from build123d import *

# Parameters (mm, degrees)
BOSS_EXTRUDE1_DEPTH = 5.08
BOSS_EXTRUDE2_DEPTH = 8.763
CHAMFER1_SIZE       = 2.54
CUT_EXTRUDE2_DEPTH  = 6.35
SKETCH6_W           = 10.16
SKETCH6_H           = 8.89
CUT_EXTRUDE3_DEPTH  = 3.81
SKETCH7_R           = 4.953
CUT_EXTRUDE4_DEPTH  = 2.54
SKETCH8_R           = 1.786664303
SKETCH8_R_2         = 1.778
CUT_EXTRUDE5_DEPTH  = 3.54
CUT_EXTRUDE6_DEPTH  = 2.54
CUT_EXTRUDE7_DEPTH  = 0.762
SKETCH11_W          = 8.89
SKETCH11_H          = 8.89
SKETCH11_R          = 1.524
BOSS_EXTRUDE3_DEPTH = 3.175


with BuildPart() as part:
    # Sketch1 → Boss-Extrude1 (new body)
    with BuildSketch(Plane.XY):
        with BuildLine():
            Line((-12.7, 0), (-12.7, -71.267258261))
            ThreePointArc((-12.7, -71.267258261), (0, -72.39), (12.7, -71.267258261))
            Line((12.7, -71.267258261), (12.7, 0))
            Line((12.7, 0), (-12.7, 0))
        make_face()
    extrude(amount=BOSS_EXTRUDE1_DEPTH)

    # Sketch4 → Boss-Extrude2 (add, symmetric)
    with BuildSketch(Plane(origin=(0, 0, 0), x_dir=(0, 0, -1), z_dir=(1, 0, 0))):
        with BuildLine():
            Line((4.336051224, -8.725020014), (0.743948776, -12.317122463))
            ThreePointArc((0.743948776, -12.317122463), (0.193345987, -13.141157769), (0, -14.113173687))
            Line((0, -14.113173687), (0, -2.54))
            Line((0, -2.54), (5.08, -4.38896879))
            Line((5.08, -4.38896879), (5.08, -6.92896879))
            ThreePointArc((5.08, -6.92896879), (4.886654013, -7.900984708), (4.336051224, -8.725020014))
        make_face()
    extrude(amount=BOSS_EXTRUDE2_DEPTH, both=True)

    # Chamfer1
    chamfer1_edges = [part.edges().sort_by_distance(p)[0] for p in [
        (0, -72.39, 0),
    ]]
    chamfer(chamfer1_edges, length=CHAMFER1_SIZE)

    # Sketch5 → Cut-Extrude2 (cut)
    with BuildSketch(Plane(origin=(0, 0, 0), x_dir=(-1, 0, 0), z_dir=(0, 0, -1))):
        with BuildLine():
            Line((-9.788025612, -42.36132736), (-5.358068299, -46.791284673))
            ThreePointArc((-5.358068299, -46.791284673), (-4.460042687, -47.163259061), (-3.562017075, -46.791284673))
            Line((-3.562017075, -46.791284673), (0.867940238, -42.36132736))
            ThreePointArc((0.867940238, -42.36132736), (1.239914626, -41.463301747), (0.867940238, -40.565276135))
            Line((0.867940238, -40.565276135), (-3.562017075, -36.135318822))
            ThreePointArc((-3.562017075, -36.135318822), (-4.460042687, -35.763344434), (-5.358068299, -36.135318822))
            Line((-5.358068299, -36.135318822), (-9.788025612, -40.565276135))
            ThreePointArc((-9.788025612, -40.565276135), (-10.16, -41.463301747), (-9.788025612, -42.36132736))
        make_face()
        with BuildLine():
            Line((-0.867940238, -33.441241986), (3.562017075, -37.871199299))
            ThreePointArc((3.562017075, -37.871199299), (4.460042687, -38.243173687), (5.358068299, -37.871199299))
            Line((5.358068299, -37.871199299), (9.788025612, -33.441241986))
            ThreePointArc((9.788025612, -33.441241986), (10.16, -32.543216374), (9.788025612, -31.645190762))
            Line((9.788025612, -31.645190762), (5.358068299, -27.215233449))
            ThreePointArc((5.358068299, -27.215233449), (4.460042687, -26.843259061), (3.562017075, -27.215233449))
            Line((3.562017075, -27.215233449), (-0.867940238, -31.645190762))
            ThreePointArc((-0.867940238, -31.645190762), (-1.239914626, -32.543216374), (-0.867940238, -33.441241986))
        make_face()
        with BuildLine():
            Line((-9.788025612, -24.521156612), (-5.358068299, -28.951113925))
            ThreePointArc((-5.358068299, -28.951113925), (-4.460042687, -29.323088313), (-3.562017075, -28.951113925))
            Line((-3.562017075, -28.951113925), (0.867940238, -24.521156612))
            ThreePointArc((0.867940238, -24.521156612), (1.239914626, -23.623131), (0.867940238, -22.725105388))
            Line((0.867940238, -22.725105388), (-3.562017075, -18.295148075))
            ThreePointArc((-3.562017075, -18.295148075), (-4.460042687, -17.923173687), (-5.358068299, -18.295148075))
            Line((-5.358068299, -18.295148075), (-9.788025612, -22.725105388))
            ThreePointArc((-9.788025612, -22.725105388), (-10.16, -23.623131), (-9.788025612, -24.521156612))
        make_face()
        with BuildLine():
            Line((-0.867940238, -51.281412733), (3.562017075, -55.711370046))
            ThreePointArc((3.562017075, -55.711370046), (4.460042687, -56.083344434), (5.358068299, -55.711370046))
            Line((5.358068299, -55.711370046), (9.788025612, -51.281412733))
            ThreePointArc((9.788025612, -51.281412733), (10.16, -50.383387121), (9.788025612, -49.485361509))
            Line((9.788025612, -49.485361509), (5.358068299, -45.055404196))
            ThreePointArc((5.358068299, -45.055404196), (4.460042687, -44.683429808), (3.562017075, -45.055404196))
            Line((3.562017075, -45.055404196), (-0.867940238, -49.485361509))
            ThreePointArc((-0.867940238, -49.485361509), (-1.239914626, -50.383387121), (-0.867940238, -51.281412733))
        make_face()
    extrude(amount=-CUT_EXTRUDE2_DEPTH, mode=Mode.SUBTRACT)

    # Sketch6 → Cut-Extrude3 (cut)
    with BuildSketch(Plane.XY.offset(5.08)):
        with Locations((0, -4.445)):
            Rectangle(SKETCH6_W, SKETCH6_H)
    extrude(amount=-CUT_EXTRUDE3_DEPTH, mode=Mode.SUBTRACT)

    # Sketch7 → Cut-Extrude4 (cut)
    with BuildSketch(Plane(origin=(0, 0, 0), x_dir=(-1, 0, 0), z_dir=(0, 0, -1))):
        with Locations((0, -67.31)):
            Circle(SKETCH7_R)
    extrude(amount=-CUT_EXTRUDE4_DEPTH, mode=Mode.SUBTRACT)

    # Sketch8 → Cut-Extrude5 (cut, through all)
    with BuildSketch(Plane(origin=(0, 0, 2.54), x_dir=(-1, 0, 0), z_dir=(0, 0, -1))):
        Circle(SKETCH8_R)
        with Locations((0, -67.31)):
            Circle(SKETCH8_R_2)
    extrude(amount=-CUT_EXTRUDE5_DEPTH, mode=Mode.SUBTRACT)

    # Sketch9 → Cut-Extrude6 (cut)
    with BuildSketch(Plane.XY.offset(5.08)):
        with BuildLine():
            Line((-12.7, -68.685751798), (-12.7, -63.51269873))
            ThreePointArc((-12.7, -63.51269873), (-9.046553162, -64.135113439), (-5.363487601, -64.547547597))
            Line((-5.363487601, -64.547547597), (-5.784153295, -69.610100349))
            ThreePointArc((-5.784153295, -69.610100349), (-9.25362555, -69.234333348), (-12.7, -68.685751798))
        make_face()
        with BuildLine():
            Line((5.784153295, -69.610100349), (5.363487601, -64.547547597))
            ThreePointArc((5.363487601, -64.547547597), (9.046553162, -64.135113439), (12.7, -63.51269873))
            Line((12.7, -63.51269873), (12.7, -68.685751798))
            ThreePointArc((12.7, -68.685751798), (9.25362555, -69.234333348), (5.784153295, -69.610100349))
        make_face()
    extrude(amount=-CUT_EXTRUDE6_DEPTH, mode=Mode.SUBTRACT)

    # Sketch10 → Cut-Extrude7 (cut)
    with BuildSketch(Plane(origin=(0, 0, 0), x_dir=(-1, 0, 0), z_dir=(0, 0, -1))):
        with BuildLine():
            Line((-10.795, -46.742506644), (-10.795, -54.024267598))
            Line((-10.795, -54.024267598), (-8.052145135, -51.281412733))
            ThreePointArc((-8.052145135, -51.281412733), (-7.680170747, -50.383387121), (-8.052145135, -49.485361509))
            Line((-8.052145135, -49.485361509), (-10.795, -46.742506644))
        make_face()
        with BuildLine():
            Line((0.867940238, -58.405446883), (-3.562017075, -53.97548957))
            ThreePointArc((-3.562017075, -53.97548957), (-4.460042687, -53.603515182), (-5.358068299, -53.97548957))
            Line((-5.358068299, -53.97548957), (-9.788025612, -58.405446883))
            ThreePointArc((-9.788025612, -58.405446883), (-10.16, -59.303472495), (-9.788025612, -60.201498107))
            Line((-9.788025612, -60.201498107), (-7.632523719, -62.357))
            Line((-7.632523719, -62.357), (-1.287561655, -62.357))
            Line((-1.287561655, -62.357), (0.867940238, -60.201498107))
            ThreePointArc((0.867940238, -60.201498107), (1.239914626, -59.303472495), (0.867940238, -58.405446883))
        make_face()
        with BuildLine():
            Line((8.052145135, -42.36132736), (10.795, -45.104182224))
            Line((10.795, -45.104182224), (10.795, -37.822421271))
            Line((10.795, -37.822421271), (8.052145135, -40.565276135))
            ThreePointArc((8.052145135, -40.565276135), (7.680170747, -41.463301747), (8.052145135, -42.36132736))
        make_face()
        with BuildLine():
            Line((-10.795, -28.902335897), (-10.795, -36.184096851))
            Line((-10.795, -36.184096851), (-8.052145135, -33.441241986))
            ThreePointArc((-8.052145135, -33.441241986), (-7.680170747, -32.543216374), (-8.052145135, -31.645190762))
            Line((-8.052145135, -31.645190762), (-10.795, -28.902335897))
        make_face()
        with BuildLine():
            Line((9.370923164, -16.018173687), (-0.45083779, -16.018173687))
            Line((-0.45083779, -16.018173687), (3.562017075, -20.031028552))
            ThreePointArc((3.562017075, -20.031028552), (4.460042687, -20.40300294), (5.358068299, -20.031028552))
            Line((5.358068299, -20.031028552), (9.370923164, -16.018173687))
        make_face()
        with BuildLine():
            Line((8.052145135, -24.521156612), (10.795, -27.264011477))
            Line((10.795, -27.264011477), (10.795, -19.982250523))
            Line((10.795, -19.982250523), (8.052145135, -22.725105388))
            ThreePointArc((8.052145135, -22.725105388), (7.680170747, -23.623131), (8.052145135, -24.521156612))
        make_face()
        with BuildLine():
            Line((8.052145135, -60.201498107), (10.207647028, -62.357))
            Line((10.207647028, -62.357), (10.795, -62.357))
            Line((10.795, -62.357), (10.795, -55.662592018))
            Line((10.795, -55.662592018), (8.052145135, -58.405446883))
            ThreePointArc((8.052145135, -58.405446883), (7.680170747, -59.303472495), (8.052145135, -60.201498107))
        make_face()
    extrude(amount=-CUT_EXTRUDE7_DEPTH, mode=Mode.SUBTRACT)

    # Sketch11 → Boss-Extrude3 (add)
    with BuildSketch(Plane.XY.offset(5.08)):
        with Locations((17.145, -27.452258261)):
            Rectangle(SKETCH11_W, SKETCH11_H)
        with Locations((17.145, -27.452258261)):
            Circle(SKETCH11_R, mode=Mode.SUBTRACT)
        with Locations((-17.145, -27.452258261)):
            Rectangle(SKETCH11_W, SKETCH11_H)
        with Locations((-17.145, -27.452258261)):
            Circle(SKETCH11_R, mode=Mode.SUBTRACT)
    extrude(amount=-BOSS_EXTRUDE3_DEPTH)


solid = part.part
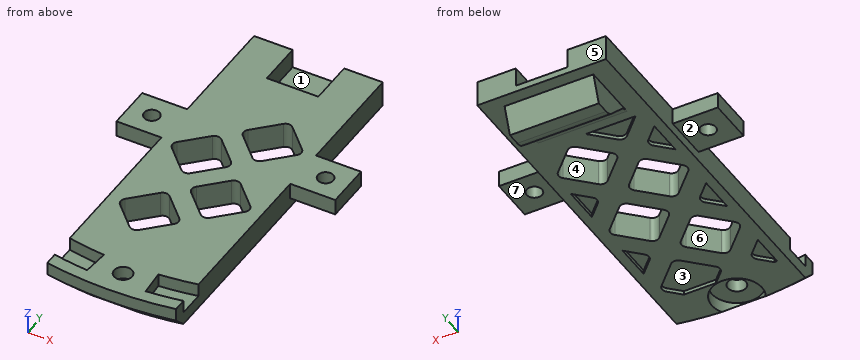
CAD build for the part. Positions are in the model's coordinates, mm. Face numbers are marked on the shaded views. A direction names the side the tool comes from. Round coordinates to 2 decimals unless told otherwise and drop trailing zeros. Write each loop counter-clockwise with the first axis right and the second up, starting at its lowest first coordinate (ties: lowest second). Pieces come first, ordered by that corner, then holes.
(1) Slice it at C-C, the plane x = 14. Write the cut outline in (y, z) (3 decimals), and give its area (3 significant figures).
(2) Probe line 1 along Y through (x, z) = (0.5, 3.5); line 2 along Y through (x, z) = (4, 2.75); line 3 along X through (y, z) = (-53, 2). List the from-to ranges inside material, lowest first.
(3) 3-axis set-ups, long thin cutter, end or side, ignore diameter. For the marked faces 1, 2, 3 and 4: which of +Z, -Z, +X, -X, +Y, -Y reach the whole face in a straight line?
(4) Slice it at D-D, the plane z = -3. Write the cut outline in (x, y).
(5) Slice it at B-B, the plane y = -6. Write the cut outline in (x, z).
(6) Slice it at A-A, the plane y = -67.31. Write the cut outline in (x, z), and give its area (3 significant figures).
(7) Drop flat-ended pins along their axis: P1, Ø4, axis at y = -23, z = -0.5, coming from the -X side; P2, Ø1.6, axis at x = 9, y = -31, coming from the -Z side; P3, Ø3, axis at x = 11, y = -66, coming from the +Z side; P4, Ø1, axis at y = -20, z = -1.5, coming from the +X side. Give the stop position or say it passes through.
(8) Mould opens along Y. For the marked faces 5, 6 and 7 say: pulls with the +Y half, pulls with the -Y half, needs draft (parallel to the pull), parting line crosses it, or undercut.
From the geometry:
1. outline: (-31.897, 1.905) - (-23.007, 1.905) - (-23.007, 5.08) - (-31.897, 5.08) - close
1. area: 28.2 mm2
2. line 1: y = -72.39 to -69.02, -65.6 to -51.65, -49.12 to -43.73, -39.2 to -33.81, -31.28 to -25.89, -21.36 to -8.89
2. line 2: y = -72.28 to -47.08, -35.85 to -29.24, -18.01 to -8.89
2. line 3: x = -12.7 to -8.07, -0.85 to 12.7
3. face 1: +Z, +Y
3. face 2: -Z, -X, +Y, -Y
3. face 3: -Z
3. face 4: +Z, -Z
4. outline: (-8.76, -10.06) - (8.76, -10.06) - (8.76, -3.63) - (-8.76, -3.63) - close
5. outline: (-12.7, 0) - (-8.76, 0) - (-8.76, -5.08) - (8.76, -5.08) - (8.76, 0) - (12.7, 0) - (12.7, 5.08) - (5.08, 5.08) - (5.08, 1.27) - (-5.08, 1.27) - (-5.08, 5.08) - (-12.7, 5.08) - close
6. outline: (-12.7, 0) - (-4.95, 0) - (-4.95, 2.54) - (-1.78, 2.54) - (-1.78, 5.08) - (-5.59, 5.08) - (-5.59, 2.54) - (-12.7, 2.54) - close; (1.78, 2.54) - (4.95, 2.54) - (4.95, 0) - (12.7, 0) - (12.7, 2.54) - (5.59, 2.54) - (5.59, 5.08) - (1.78, 5.08) - close
6. area: 58.7 mm2
7. P1: stops at x = -12.7
7. P2: stops at z = 0
7. P3: stops at z = 2.54
7. P4: passes through
8. face 5: pulls with the +Y half
8. face 6: undercut
8. face 7: needs draft
